```python
from build123d import *

# Parameters (mm, degrees)
F0_W     = 35
F0_H     = 55
F1_DEPTH = 30
F3_W     = 23
F3_H     = 44
F4_DEPTH = 40
F6_D     = 10


with BuildPart() as f1:
    # F0 (on Top) → F1 (new body)
    with BuildSketch(Plane.XY):
        Rectangle(F0_W, F0_H)
    extrude(amount=F1_DEPTH)

    # F3 (on face) → F4 (cut)
    with BuildSketch(Plane.XY.offset(30)):
        Rectangle(F3_W, F3_H)
    extrude(amount=-F4_DEPTH, mode=Mode.SUBTRACT)

    # F6 (through all)
    with Locations(Plane.YZ.offset(17.5)):
        with Locations((0, 15)):
            Hole(F6_D / 2)


solid = f1.part
```
Check sheet for the modelled part. Datum: model origin and axes. Units: mm. A direction names the side the tool comes from. Give positions to 0.01 mm unless a question says otherwise; leave off trailing zeros. Order: outer loops, then holes, each group sorted by start corner. A loop starts at its lowest first (then second) coordinate and runs counter-clockwise, first axis right, second up. Notation, with made-up numbers: M 52,85.25 L 87,85.25 A35 ccw 87,121.25 Z; hole C 26.5,-8.5 d8. An arc over 180 degrees is marked long. Answer in a Markdown table with one row per item. Add a question column.
Q1. Release check for a two-part mould opening along Z. For faces 1 (the cylindrical face through (-14.54, 1.08, 10.12)), 2 (the flat face through (-12, 0, 30)), 3 (the flat face through (0, -22, 15)), 4 (the cylindrical face through (14.46, 1.08, 10.12)) record: released by +Z, released by -Z, zero draft, split by the parting line, or undercut.
Q2. Access from +Z, -Z, +X, -X, +Y, -Y to the whole of each face (thin tool, end or side, straight path). Record for faces 5 (the flat face through (0, -27.5, 15)), 6 (the flat face through (11.5, -5.2, 15.2)).
Q3. Gauge pin test, flat ends, axial feed: pin 1 Ø4 at (x, y) = (-8, 0) entering from +Z; pin 2 Ø1.5 at (x, y) = (-12.5, -4.5) entering from -Z. Record the tip position at first contact, or that the pin passes through.
Q4. Sectioned sample at A-A, the plane y = 0. Record the boundary of the cut face in (x, z).
Q5. Thickness scan on L1, parallel to X at y = 21, z = 24.5; L2, parallel to Z at x = 12.85, y = 0; L3, parallel to Y at x = -11, z = 2.75. Record the ranges inside material, lowest first.
Q6. Sectioned sample at B-B, the plane x = -5. Record the boundary of the cut face in (y, z), and give its area (3 significant figures).
Q7. Sectioned sample at C-C, the plane y = 8.5. Record the boundary of the cut face in (x, z), and give its area (3 significant figures).
Q8. Sectioned sample at D-D, the plane z = 15. Record the boundary of the cut face in (x, y).
Verdict:
| question | item | result |
|---|---|---|
| 1 | face 1 | undercut |
| 1 | face 2 | released by +Z |
| 1 | face 3 | zero draft |
| 1 | face 4 | undercut |
| 2 | face 5 | +Z, -Z, +X, -X, -Y |
| 2 | face 6 | +Z, -Z |
| 3 | pin 1 | through |
| 3 | pin 2 | z = 0 |
| 4 | outline | M -17.5,0 L -11.5,0 L -11.5,10 L -17.5,10 Z; M -17.5,20 L -11.5,20 L -11.5,30 L -17.5,30 Z; M 11.5,0 L 17.5,0 L 17.5,10 L 11.5,10 Z; M 11.5,20 L 17.5,20 L 17.5,30 L 11.5,30 Z |
| 5 | L1 | -17.5 to -11.5, 11.5 to 17.5 |
| 5 | L2 | 0 to 10, 20 to 30 |
| 5 | L3 | -27.5 to -22, 22 to 27.5 |
| 6 | outline | M -27.5,0 L -22,0 L -22,30 L -27.5,30 Z; M 22,0 L 27.5,0 L 27.5,30 L 22,30 Z |
| 6 | area | 330 mm² |
| 7 | outline | M -17.5,0 L -11.5,0 L -11.5,30 L -17.5,30 Z; M 11.5,0 L 17.5,0 L 17.5,30 L 11.5,30 Z |
| 7 | area | 360 mm² |
| 8 | outline | M -17.5,-27.5 L 17.5,-27.5 L 17.5,-5 L 11.5,-5 L 11.5,-22 L -11.5,-22 L -11.5,-5 L -17.5,-5 Z; M -17.5,5 L -11.5,5 L -11.5,22 L 11.5,22 L 11.5,5 L 17.5,5 L 17.5,27.5 L -17.5,27.5 Z |
